For this review, take the finished solid that the model builds, in its own axes (mm). Give positions to 0.01 mm unless a question says otherwise; leave off trailing zeros.
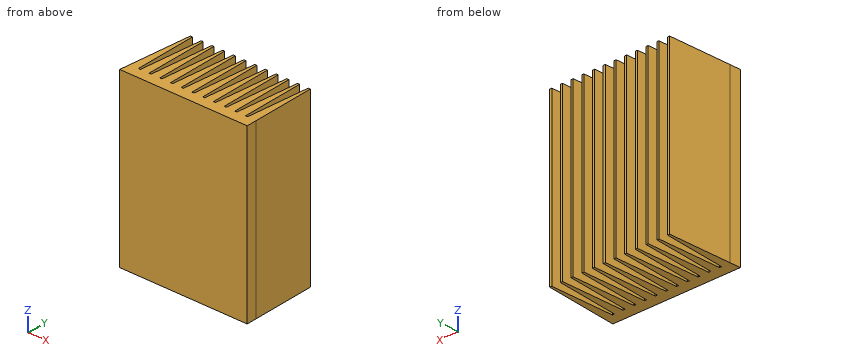
from build123d import *

# Parameters (mm, degrees)
BOSS_EXTRUDE1_DEPTH = 80


with BuildPart() as part:
    # Sketch2 → Boss-Extrude1 (new body)
    with BuildSketch(Plane.XY):
        Polygon((-20.657894737, -2.5), (20.657894737, -2.5), (20.39585584, 2.5), (18.823622462, 32.5), (17.823622462, 32.5), (16.251389083, 2.5), (15.251389083, 2.5), (13.679155705, 32.5), (12.679155705, 32.5), (11.106922326, 2.5), (10.106922326, 2.5), (8.534688948, 32.5), (7.534688948, 32.5), (5.962455569, 2.5), (4.962455569, 2.5), (3.390222191, 32.5), (2.390222191, 32.5), (0.817988812, 2.5), (-0.182011188, 2.5), (-1.754244566, 32.5), (-2.754244566, 32.5), (-4.326477944, 2.5), (-5.326477944, 2.5), (-6.898711323, 32.5), (-7.898711323, 32.5), (-9.470944701, 2.5), (-10.470944701, 2.5), (-12.04317808, 32.5), (-13.04317808, 32.5), (-14.615411458, 2.5), (-15.615411458, 2.5), (-17.187644837, 32.5), (-18.187644837, 32.5), (-19.759878215, 2.5), (-20.759878215, 2.5), (-22.332111594, 32.5), (-23.332111594, 32.5), (-24.904344972, 2.5), (-25.904344972, 2.5), (-27.476578351, 32.5), (-28.476578351, 32.5), (-30.048811729, 2.5), (-31.048811729, 2.5), (-32.621045108, 32.5), (-33.621045108, 32.5), (-35.193278486, 2.5), (-36.193278486, 2.5), (-37.765511865, 32.5), (-38.765511865, 32.5), (-40.337745243, 2.5), (-40.59978414, -2.5), align=None)
    extrude(amount=BOSS_EXTRUDE1_DEPTH)


solid = part.part
1) We need section A-A on y = 23.5. Count the separate pieces of the cut face and the enclosed holes in it, then the cut area to 3 significant figures.
Answer sheet:
separate pieces: 12
enclosed holes: 0
area: 1,870 mm2
2) To check wall thickness, follow line 1 (Y direction, x = 16, z = 59). State the ranges of the line that lie inside material, in increasing order.
Answer sheet:
line 1: y = -2.5 to 2.5
3) Clearance check with flat-ended pins moving along their axes: pin 1 (0.5 mm diameter, centred on x = -25.5, z = 33.5, fed in from +Y); pin 2 (2 mm diameter, centred on y = 2.5, z = 28, fed in from -X). State where each tip first meets the part, or that it passes through.
Answer sheet:
pin 1: stops at y = 2.5
pin 2: stops at x = -40.39
